The listing builds one solid part. Answer for the finished solid, in the listing's coordinates (mm). Round coordinates to 2 decimals unless told otherwise and drop trailing zeros. Write each loop counter-clockwise with the first axis right and the second up, starting at its lowest first coordinate (ties: lowest second). Pieces come first, ordered by that corner, then holes. Notation, with made-up numbers: M 22.25,-1.75 L 76.25,-1.75 A19 ccw 76.25,14.25 Z; hole C 24.5,11 d5. An arc over 180 degrees is marked long. Put each result on its own line as item: value. Start each with the question number.
```python
from build123d import *

# Parameters (mm, degrees)
SKETCH1_W           = 38.1
SKETCH1_H           = 38.1
BOSS_EXTRUDE1_DEPTH = 3.175
SKETCH2_R           = 1.5
CUT_EXTRUDE1_DEPTH  = 4.175
SKETCH3_R           = 3.175
CUT_EXTRUDE2_DEPTH  = 4.175


with BuildPart() as part:
    # Sketch1 → Boss-Extrude1 (new body)
    with BuildSketch(Plane(origin=(0, 0, 0), x_dir=(1, 0, 0), z_dir=(0, 1, 0))):
        Rectangle(SKETCH1_W, SKETCH1_H)
    extrude(amount=BOSS_EXTRUDE1_DEPTH)

    # Sketch2 → Cut-Extrude1 (cut, through all)
    with BuildSketch(Plane(origin=(0, 3.175, 0), x_dir=(1, 0, 0), z_dir=(0, 1, 0))):
        with Locations((0, 7.5)):
            Circle(SKETCH2_R)
        with Locations((6.495190528, -3.75)):
            Circle(SKETCH2_R)
        with Locations((-6.495190528, -3.75)):
            Circle(SKETCH2_R)
    extrude(amount=-CUT_EXTRUDE1_DEPTH, mode=Mode.SUBTRACT)

    # Sketch3 → Cut-Extrude2 (cut, through all)
    with BuildSketch(Plane(origin=(0, 3.175, 0), x_dir=(1, 0, 0), z_dir=(0, 1, 0))):
        with Locations((-12.7, 12.7)):
            Circle(SKETCH3_R)
        with Locations((-12.7, -12.7)):
            Circle(SKETCH3_R)
        with Locations((12.7, -12.7)):
            Circle(SKETCH3_R)
        with Locations((12.7, 12.7)):
            Circle(SKETCH3_R)
    extrude(amount=-CUT_EXTRUDE2_DEPTH, mode=Mode.SUBTRACT)


solid = part.part
```
Item 1: Section B-B (y = 0.95) is taken. Give the vertices of the cut face in (x, z) (3 decimals).
Item 2: Determine the mould class of faces 1 (the flat face through (19.05, 2, 0)), 2 (the flat face through (0, 3.175, 0)), 3 (the cylindrical face through (7.302, 1.61, 2.485)) for opening direction X: released by +X, released by -X, zero draft, split by the parting line, or undercut.
Item 3: Section A-A (z = 3.75) is taken. Give the vertices of the cut face in (x, y) (3 decimals), and give its area (3 significant figures).
Item 4: Consider line 1 along X through (y, z) = (1, 3.75); line 2 along X through (y, z) = (2.05, -12.7) (3 decimals). Determine where each line is inside the solid, lowest interval first. Write a range as [from, to].
Item 5: Section D-D (z = -7.5) is taken. Give the vertices of the cut face in (x, y) (3 decimals), and give its area (3 significant figures).
Item 6: Section C-C (x = 0) is taken. Give the vertices of the cut face in (y, z) (3 decimals).
Output values:
1. outline: M -19.05,-19.05 L 19.05,-19.05 L 19.05,19.05 L -19.05,19.05 Z; hole C -12.7,-12.7 d6.35; hole C -12.7,12.7 d6.35; hole C -6.495,3.75 d3; hole C 0,-7.5 d3; hole C 6.495,3.75 d3; hole C 12.7,-12.7 d6.35; hole C 12.7,12.7 d6.35
2. face 1: released by +X
2. face 2: zero draft
2. face 3: undercut
3. outline: M -19.05,0 L -7.995,0 L -7.995,3.175 L -19.05,3.175 Z; M -4.995,0 L 4.995,0 L 4.995,3.175 L -4.995,3.175 Z; M 7.995,0 L 19.05,0 L 19.05,3.175 L 7.995,3.175 Z
3. area: 102 mm^2
4. line 1: x = [-19.05, -8], [-5, 5], [8, 19.05]
4. line 2: x = [-19.05, -15.875], [-9.525, 9.525], [15.875, 19.05]
5. outline: M -19.05,0 L -1.5,0 L -1.5,3.175 L -19.05,3.175 Z; M 1.5,0 L 19.05,0 L 19.05,3.175 L 1.5,3.175 Z
5. area: 111 mm^2
6. outline: M 0,-19.05 L 3.175,-19.05 L 3.175,-9 L 0,-9 Z; M 0,-6 L 3.175,-6 L 3.175,19.05 L 0,19.05 Z
